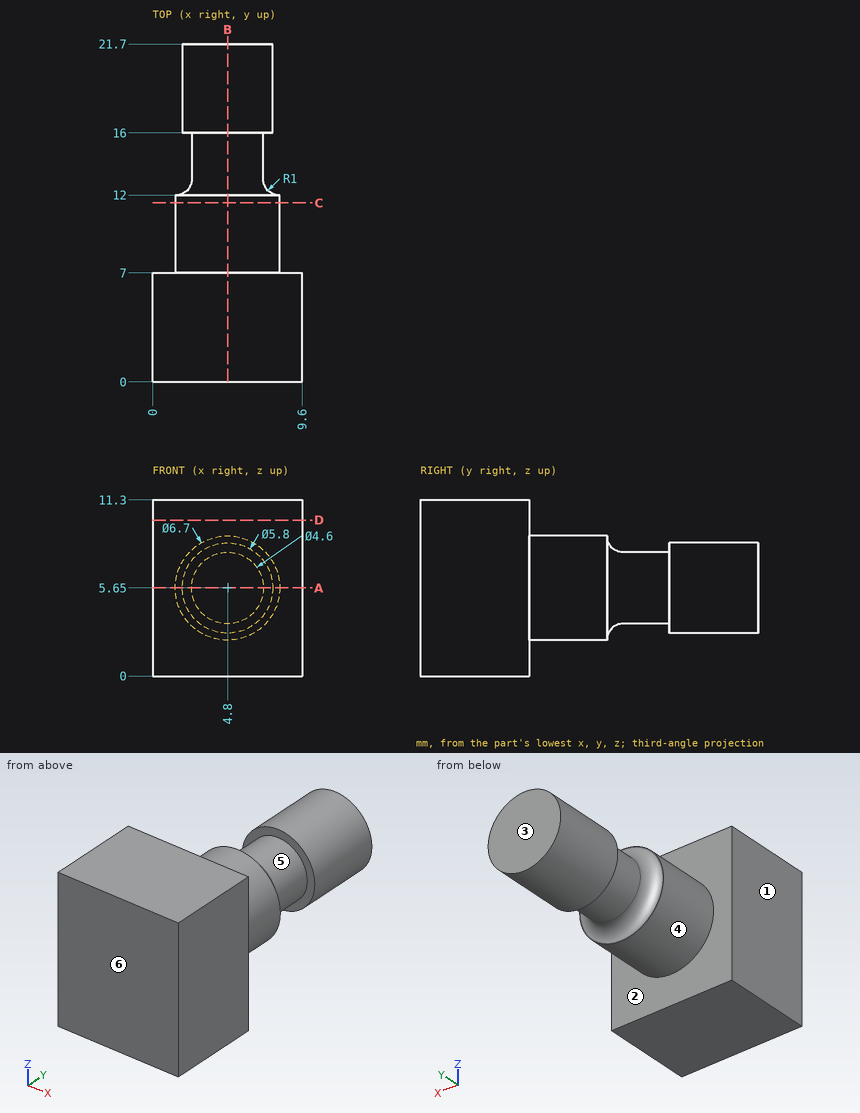
Verification items for this drawing (mm, ordinates from the low corner). A direction names the side the tool comes from. Coordinates: 2 decimals unless noted, no trailing zeros. Loops run counter-clockwise (first coordinate to the right, second up) from the corner with the lowest first, then second, coordinate; pieces in that order, holes last. Notation, with made-up numbers: (82, 57) - (111, 57) arc R18 cw to (111, 81) - close; hole circle Ø5 at (39, 33). An arc over 180 degrees is marked (long way). Answer as a JSON object with one key per item and string values.
(1) Scan lines: line 1 along Y through (x, z) = (6.5, 1.75); line 2 along Y through (x, z) = (5.5, 8.25); line 3 along X through (y, z) = (19.75, 5.5). Record each from-to range of solid material in increasing order.
Response:
{"line 1": "y = 0 to 7", "line 2": "y = 0 to 12.21, 16 to 21.7", "line 3": "x = 1.9 to 7.7"}
(2) Cross-section at A-A, the plane z = 5.65. Record the boundary of the cut face in (x, y).
Response:
{"outline": "(0, 0) - (9.6, 0) - (9.6, 7) - (8.15, 7) - (8.15, 12) - (8.1, 12) arc R1 cw to (7.1, 13) - (7.1, 16) - (7.7, 16) - (7.7, 21.7) - (1.9, 21.7) - (1.9, 16) - (2.5, 16) - (2.5, 13) arc R1 cw to (1.5, 12) - (1.45, 12) - (1.45, 7) - (0, 7) - close"}
(3) Cross-section at D-D, the plane z = 10. Record the boundary of the cut face in (x, y), then the cut area to 3 significant figures.
Response:
{"outline": "(0, 0) - (9.6, 0) - (9.6, 7) - (0, 7) - close", "area": "67.2 mm²"}
(4) Go/stop test with flat-tipped pins: pin 1 Ø4 at (x, z) = (1.5, 9.5) entering from +Y; pin 2 Ø1 at (x, y) = (5.5, 10) entering from +Z; pin 3 Ø1 at (x, y) = (2.5, 13.5) entering from -Z. Record where each tip stops, or that it passes through.
Response:
{"pin 1": "stops at y = 12.03", "pin 2": "stops at z = 8.99", "pin 3": "stops at z = 4.22"}
(5) Access from +Z, -Z, +X, -X, +Y, -Y to the whole of each face (thin tool, end or side, straight path). Record for the marked faces 1 and 2.
Response:
{"face 1": "+Z, -Z, -X, +Y, -Y", "face 2": "+Y"}
(6) Mould release check, pull along Y, two halves, no side actions. Record for the marked faces 3, 4, 5 and 6: pulls with the +Y half, pulls with the -Y half, needs draft (parallel to the pull), parting line crosses it, or undercut.
Response:
{"face 3": "pulls with the +Y half", "face 4": "needs draft", "face 5": "undercut", "face 6": "pulls with the -Y half"}
(7) Cross-section at C-C, the plane y = 11.5. Record the boundary of the cut face in (x, z), then the cut area to 3 significant figures.
Response:
{"outline": "circle Ø6.7 at (4.8, 5.65)", "area": "35.3 mm²"}
(8) Cross-section at B-B, the plane x = 4.8. Record the boundary of the cut face in (y, z), then the cut area to 3 significant figures.
Response:
{"outline": "(0, 0) - (7, 0) - (7, 2.3) - (12, 2.3) - (12, 2.35) arc R1 cw to (13, 3.35) - (16, 3.35) - (16, 2.75) - (21.7, 2.75) - (21.7, 8.55) - (16, 8.55) - (16, 7.95) - (13, 7.95) arc R1 cw to (12, 8.95) - (12, 9) - (7, 9) - (7, 11.3) - (0, 11.3) - close", "area": "164 mm²"}
